Geometry check sheet. Reference: drawing and pictorial views, mm from the part's lowest x, y, z. Give positions to 0.01 mm unless a question says otherwise; leave off trailing zeros. Write each loop counter-clockwise with the first axis right and the second up, starting at its lowest first coordinate (ties: lowest second). Pieces come first, ordered by that corner, then holes. Notation, with made-up numbers: (0, 83.5) -> (51, 83.5) arc R29 cw to (51, 119.5) -> close; hole circle Ø9 at (20, 30). An arc over 180 degrees is marked (long way). Use a Markdown table: item, result. Add a question column.
1. Cross-section at A-A (x = 12). Enter the section's corners in (y, z).
2. Cross-section at B-B (z = 32). Enter the section's corners in (x, y), then the cut area to 3 significant figures.
3. Gauge pin test, flat ends, axial feed: P1, Ø0.9, axis at y = 0, z = 36.5, coming from the -X side; P2, Ø0.9, axis at y = 0.5, z = 38, coming from the +X side; P3, Ø3, axis at x = 12, z = 2, coming from the +Y side. Record the tip position at first contact, or that the pin passes through.
4. Cross-section at D-D (z = 26.5). Enter the section's corners in (x, y), then the cut area to 3 significant figures.
5. Cross-section at C-C (x = 8). Enter the section's corners in (y, z).
6. Scan lines: probe 1 along X at (y, z) = (0.2, 32); probe 2 along Z at (x, y) = (15.75, 0.7); probe 3 along Y at (x, z) = (11, 9). Record each from-to range of solid material in increasing order. Write a range as [from, to].
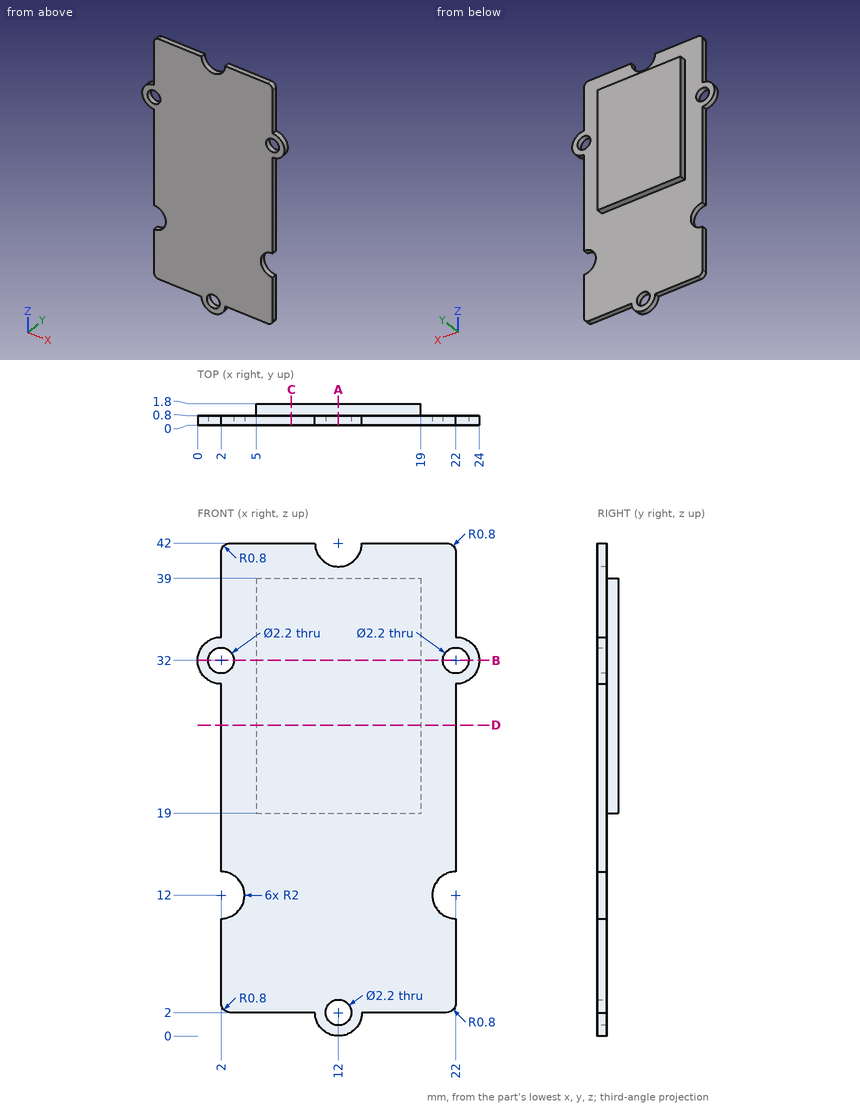
Worked answers:
| question | item | result |
|---|---|---|
| 1 | outline | (0, 0) -> (0.8, 0) -> (0.8, 0.9) -> (0, 0.9) -> close; (0, 3.1) -> (0.8, 3.1) -> (0.8, 19) -> (1.8, 19) -> (1.8, 39) -> (0.8, 39) -> (0.8, 40) -> (0, 40) -> close |
| 2 | outline | (0, 0) -> (0.9, 0) -> (0.9, 0.8) -> (0, 0.8) -> close; (3.1, 0) -> (20.9, 0) -> (20.9, 0.8) -> (19, 0.8) -> (19, 1.8) -> (5, 1.8) -> (5, 0.8) -> (3.1, 0.8) -> close; (23.1, 0) -> (24, 0) -> (24, 0.8) -> (23.1, 0.8) -> close |
| 2 | area | 29.7 mm² |
| 3 | P1 | stops at x = 2 |
| 3 | P2 | stops at x = 22 |
| 3 | P3 | stops at y = 0.8 |
| 4 | outline | (2, 0) -> (22, 0) -> (22, 0.8) -> (19, 0.8) -> (19, 1.8) -> (5, 1.8) -> (5, 0.8) -> (2, 0.8) -> close |
| 4 | area | 30.0 mm² |
| 5 | outline | (0, 2) -> (0.8, 2) -> (0.8, 19) -> (1.8, 19) -> (1.8, 39) -> (0.8, 39) -> (0.8, 42) -> (0, 42) -> close |
| 6 | probe 1 | x = [0, 0.9], [3.1, 20.9], [23.1, 24] |
| 6 | probe 2 | z = [2, 42] |
| 6 | probe 3 | y = [0, 0.8] |
